Part print with two shaded views. Sizes in mm from the minimum x, y, z corner. Round coordinates to 2 decimals unless told otherwise and drop trailing zeros. Order: outer loops, then holes, each group sorted by start corner. A loop starts at its lowest first (then second) coordinate and runs counter-clockwise, first axis right, second up. Notation, with made-up numbers: (-37, -27.5) - (-7, -27.5) arc R24 cw to (-7, -15.5) - close; hole circle Ø5 at (47, -28). An arc over 180 degrees is marked (long way). Write item = value, one per line.
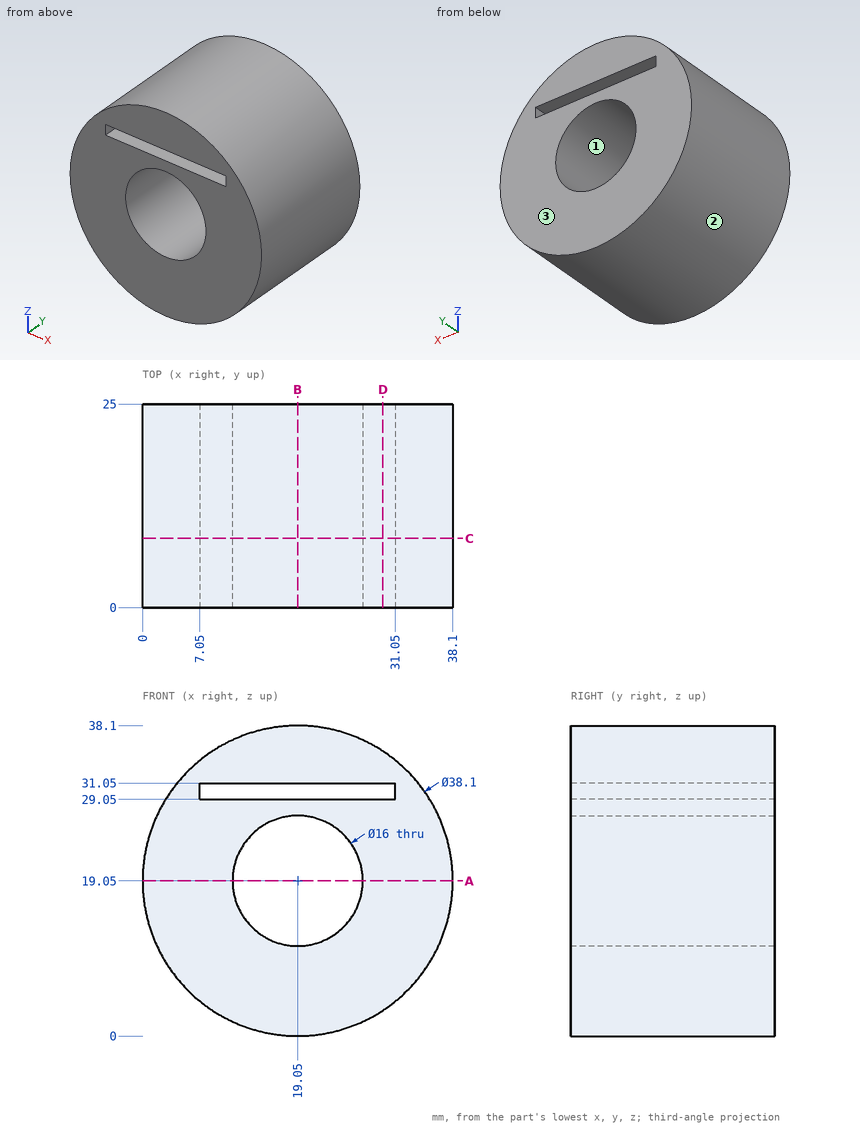
1) Wall check: line 1 along Z through (x, y) = (19.05, 7); line 2 along Z through (x, y) = (25.5, 3); line 3 along Z through (x, y) = (10, 12.75). Give the ranges that are in metal, low to high.
Conclusion:
line_1 = 0 to 11.05, 27.05 to 29.05, 31.05 to 38.1
line_2 = 1.13 to 14.32, 23.78 to 29.05, 31.05 to 36.97
line_3 = 2.29 to 29.05, 31.05 to 35.81
2) Flat gauge pins, fed straight in: pin 1 Ø1 at (y, z) = (16.5, 29.5) entering from -X (3 decimals); pin 2 Ø12 at (x, y) = (25, 13) entering from +Z; pin 3 Ø12 at (y, z) = (6.5, 5.5) entering from -X. Where does each tip first touch, or does it go through?
Conclusion:
pin_1 = 2.805
pin_2 = 38.1
pin_3 = 1.56
3) Cut at A-A (z = 19.05). Write the cut outline in (x, y).
Conclusion:
outline = (0, 0) - (11.05, 0) - (11.05, 25) - (0, 25) - close; (27.05, 0) - (38.1, 0) - (38.1, 25) - (27.05, 25) - close
4) Cut at D-D (x = 29.5). Write the cut outline in (y, z), and give its area (3 significant figures).
Conclusion:
outline = (0, 3.12) - (25, 3.12) - (25, 29.05) - (0, 29.05) - close; (0, 31.05) - (25, 31.05) - (25, 34.98) - (0, 34.98) - close
area = 746 mm^2
5) Mould opens along Z. For the marked faces 1, 2 and 3 say: +Z half, -Z half, draft (parallel to the pull), parting line (faces both ways), or undercut.
Conclusion:
face_1 = undercut
face_2 = parting line
face_3 = draft
6) Cut at B-B (x = 19.05). Write the cut outline in (y, z), and give its area (4 significant figures).
Conclusion:
outline = (0, 0) - (25, 0) - (25, 11.05) - (0, 11.05) - close; (0, 27.05) - (25, 27.05) - (25, 29.05) - (0, 29.05) - close; (0, 31.05) - (25, 31.05) - (25, 38.1) - (0, 38.1) - close
area = 502.5 mm^2
7) Cut at C-C (y = 8.5). Write the cut outline in (x, z).
Conclusion:
outline = circle Ø38.1 at (19.05, 19.05); hole (7.05, 29.05) - (31.05, 29.05) - (31.05, 31.05) - (7.05, 31.05) - close; hole circle Ø16 at (19.05, 19.05)
